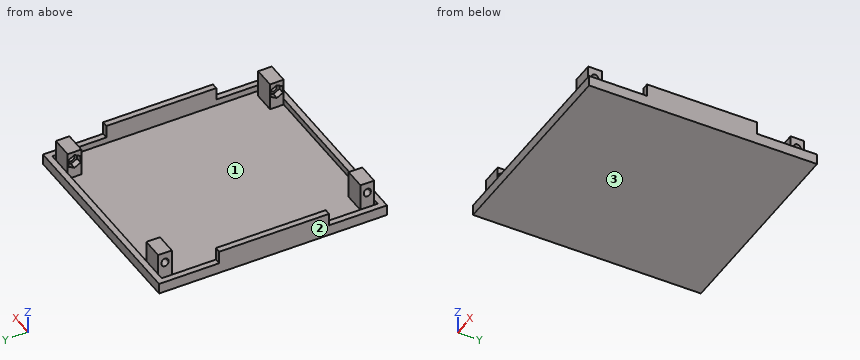
from build123d import *

# Parameters (mm, degrees)
SKETCH017_W     = 98
SKETCH017_H     = 107
PAD015_DEPTH    = 5
SKETCH018_W     = 92.4
SKETCH018_H     = 101.4
POCKET_DEPTH    = 3
SKETCH019_W     = 2.8
SKETCH019_H     = 51.6
PAD016_DEPTH    = 6
SKETCH020_W     = 10
SKETCH020_H     = 6.4
PAD017_DEPTH    = 13
POCKET001_DEPTH = 92.201
POCKET019_DEPTH = 3
POCKET020_DEPTH = 3


with BuildPart() as part:
    # Sketch017 → Pad015 (new body)
    with BuildSketch(Plane.XY.offset(-22)):
        with Locations((0.5, 0.5)):
            Rectangle(SKETCH017_W, SKETCH017_H)
    extrude(amount=PAD015_DEPTH)

    # Sketch018 (on Face6 of Pad015) → Pocket (cut)
    with BuildSketch(Plane.XY.offset(-17)):
        with Locations((0.5, 0.5)):
            Rectangle(SKETCH018_W, SKETCH018_H)
    extrude(amount=-POCKET_DEPTH, mode=Mode.SUBTRACT)

    # Sketch019 (on Face5 of Pocket) → Pad016 (join)
    with BuildSketch(Plane.XY.offset(-17)):
        with Locations((-47.1, 0)):
            Rectangle(SKETCH019_W, SKETCH019_H)
        with Locations((48.1, 0)):
            Rectangle(SKETCH019_W, SKETCH019_H)
    extrude(amount=PAD016_DEPTH)

    # Sketch020 (on Face21 of Pad016) → Pad017 (join)
    with BuildSketch(Plane.XY.offset(-20)):
        with Locations((-37.7, 48)):
            Rectangle(SKETCH020_W, SKETCH020_H)
        with Locations((38.7, 48)):
            Rectangle(SKETCH020_W, SKETCH020_H)
        with Locations((-37.7, -47)):
            Rectangle(SKETCH020_W, SKETCH020_H)
        with Locations((38.7, -47)):
            Rectangle(SKETCH020_W, SKETCH020_H)
    extrude(amount=PAD017_DEPTH)

    # Sketch021 (on Face37 of Pad017) → Pocket001 (cut, through all)
    with BuildSketch(Plane.YZ.offset(43.7)):
        with BuildLine():
            ThreePointArc((-45.4, -11.6), (-47, -10), (-48.6, -11.6))
            Line((-48.6, -11.6), (-48.6, -12.4))
            ThreePointArc((-48.6, -12.4), (-47, -14), (-45.4, -12.4))
            Line((-45.4, -11.6), (-45.4, -12.4))
        make_face()
        with BuildLine():
            ThreePointArc((49.6, -11.6), (48, -10), (46.4, -11.6))
            Line((46.4, -11.6), (46.4, -12.4))
            ThreePointArc((46.4, -12.4), (48, -14), (49.6, -12.4))
            Line((49.6, -11.6), (49.6, -12.4))
        make_face()
    extrude(amount=-POCKET001_DEPTH, mode=Mode.SUBTRACT)

    # Sketch055 (on Face40 of Pocket001) → Pocket019 (cut)
    with BuildSketch(Plane.YZ.offset(-32.7)):
        Polygon((-49.9, -13.674316), (-47, -15.348632), (-44.1, -13.674316), (-44.1, -10.325684), (-47, -8.651368), (-49.9, -10.325684), align=None)
        Polygon((48, -15.348632), (50.9, -13.674316), (50.9, -10.325684), (48, -8.651368), (45.1, -10.325684), (45.1, -13.674316), align=None)
    extrude(amount=-POCKET019_DEPTH, mode=Mode.SUBTRACT)

    # Sketch056 (on Face39 of Pocket019) → Pocket020 (cut)
    with BuildSketch(Plane(origin=(33.7, 0, 0), x_dir=(0, -1, 0), z_dir=(-1, 0, 0))):
        Polygon((47, -15.348632), (49.9, -13.674316), (49.9, -10.325684), (47, -8.651368), (44.1, -10.325684), (44.1, -13.674316), align=None)
        Polygon((-45.1, -13.674316), (-45.1, -10.325684), (-48, -8.651368), (-50.9, -10.325684), (-50.9, -13.674316), (-48, -15.348632), align=None)
    extrude(amount=-POCKET020_DEPTH, mode=Mode.SUBTRACT)


solid = part.part
Input: part model. Units: mm. Frame: model coordinates. Face numbers are marked on the shaded views. Coordinates: 2 decimals unless noted, no trailing zeros. Write each loop counter-clockwise with the first axis right and the second up, starting at its lowest first coordinate (ties: lowest second). Pieces come first, ordered by that corner, then holes. Notation, with made-up numbers: M 34,73.5 L 39,73.5 A11 cw 39,79.5 Z; hole C 77,89 d3. An arc over 180 degrees is marked long. Answer as a JSON object with one key per item and string values. Group by question number.
(1) Contact query for flat-ended pins moving along their axis: P1, Ø3, axis at x = -37, z = -15, coming from the +Y side; P2, Ø0.8, axis at x = 48.5, z = -13.5, coming from the +Y side; P3, Ø6, axis at x = -35.5, y = 3.5, coming from the +Z side; P4, Ø8, axis at x = -27.5, z = -9, coming from the +Y side. Output: stop coordinate, or through.
(2) Section B-B on y = -32.5. Output: boundary loops of the cut face in (x, z), plus the area to 3 significant figures.
(3) Ray query, line 1 along X through (y, z) = (43.5, -19); line 2 along Y through (x, z) = (26, -18); line 3 along Y through (x, z) = (-37.5, -18). Return the intervals inside material, ascending. Write a range as [from, to].
(4) Mould query, pull axis X, two halves, no side actions, for the marked faces 1, 2 and 3. Classes: pulls with the +X half, pulls with the -X half, needs draft (parallel to the pull), parting line crosses it, or undercut.
(5) Section A-A on x = -18. Output: boundary loops of the cut face in (y, z), plus the area to 3 significant figures.
Result set:
{
 "1": {"P1": "stops at y = 51.2", "P2": "stops at y = 25.8", "P3": "stops at z = -20", "P4": "passes through"},
 "2": {"outline": "M -48.5,-22 L 49.5,-22 L 49.5,-17 L 46.7,-17 L 46.7,-20 L -45.7,-20 L -45.7,-17 L -48.5,-17 Z", "area": "213 mm2"},
 "3": {"line 1": "x = [-48.5, -45.7], [46.7, 49.5]", "line 2": "y = [-53, -50.2], [51.2, 54]", "line 3": "y = [-53, -43.8], [44.8, 54]"},
 "4": {"face 1": "undercut", "face 2": "pulls with the -X half", "face 3": "needs draft"},
 "5": {"outline": "M -53,-22 L 54,-22 L 54,-17 L 51.2,-17 L 51.2,-20 L -50.2,-20 L -50.2,-17 L -53,-17 Z", "area": "231 mm2"}
}
